Here's how the part is built. I have some questions about the finished solid (model axes, mm). A direction names the side the tool comes from. Coordinates: 2 decimals unless noted, no trailing zeros. Order: outer loops, then holes, each group sorted by start corner. A loop starts at its lowest first (then second) coordinate and runs counter-clockwise, first axis right, second up. Notation, with made-up numbers: (52.5, -37.75) - (91.5, -37.75) arc R8 cw to (91.5, -22.75) - close; hole circle Ø11 at (15, -1.75). An arc over 180 degrees is marked (long way). Use one line per item in the form item = value. Start each with the question number.
from build123d import *

# Parameters (mm, degrees)
SKETCH_1_W          = 55
SKETCH_1_H          = 55
EXTRUDE_1_DEPTH     = 10
EXTRUDE_2_DEPTH     = 55
CUT_EXTRUDE_1_DEPTH = 50
SKETCH_4_R          = 3
CUT_EXTRUDE_2_DEPTH = 10
SKETCH_5_R          = 1.5
CUT_EXTRUDE_3_DEPTH = 30


with BuildPart() as part:
    # 草图1 → 凸台-拉伸1 (new body)
    with BuildSketch(Plane.XY):
        Rectangle(SKETCH_1_W, SKETCH_1_H)
    extrude(amount=EXTRUDE_1_DEPTH)

    # 草图2 → 凸台-拉伸2 (add)
    with BuildSketch(Plane(origin=(27.5, 0, 0), x_dir=(0, 0, -1), z_dir=(1, 0, 0))):
        Polygon((0, -27.5), (-14.219889521, -52.26914509), (-61.918339647, -24.885612528), (-10, 27.5), align=None)
    extrude(amount=-EXTRUDE_2_DEPTH)

    # 草图3 → 切除-拉伸1 (cut)
    with BuildSketch(Plane(origin=(0, 0, 10), x_dir=(-1, 0, 0), z_dir=(0, 0, -1))):
        Polygon((22.5, 22.5), (22.5, -22.5), (-22.5, -22.5), (-22.5, 22.5), (-22.5, 36.625124929), (22.5, 36.625124929), align=None)
    extrude(amount=-CUT_EXTRUDE_1_DEPTH, mode=Mode.SUBTRACT)

    # 草图4 → 切除-拉伸2 (cut)
    with BuildSketch(Plane(origin=(0, 0, 0), x_dir=(-1, 0, 0), z_dir=(0, 0, -1))):
        with Locations((16, 0)):
            Circle(SKETCH_4_R)
        with Locations((11.313708499, -11.313708499)):
            Circle(SKETCH_4_R)
        with Locations((0, -16)):
            Circle(SKETCH_4_R)
        with Locations((-11.313708499, -11.313708499)):
            Circle(SKETCH_4_R)
        with Locations((-16, 0)):
            Circle(SKETCH_4_R)
        with Locations((-11.313708499, 11.313708499)):
            Circle(SKETCH_4_R)
        with Locations((0, 16)):
            Circle(SKETCH_4_R)
        with Locations((11.313708499, 11.313708499)):
            Circle(SKETCH_4_R)
    extrude(amount=-CUT_EXTRUDE_2_DEPTH, mode=Mode.SUBTRACT)

    # 草图5 → 切除-拉伸3 (cut)
    with BuildSketch(Plane(origin=(0, -45.452255494, 26.093999177), x_dir=(1, 0, 0), z_dir=(0, -0.8672445477434421, 0.4978824102228085))):
        with Locations(Location((10, 23.808233719, 0), (0, 0, 270))):
            Circle(SKETCH_5_R)
        with Locations(Location((10, 13.808233719, 0), (0, 0, 270))):
            Circle(SKETCH_5_R)
        with Locations(Location((0, 23.808233719, 0), (0, 0, 270))):
            Circle(SKETCH_5_R)
        with Locations(Location((-10, 23.808233719, 0), (0, 0, 90))):
            Circle(SKETCH_5_R)
        with Locations(Location((-10, 13.808233719, 0), (0, 0, 90))):
            Circle(SKETCH_5_R)
        with Locations(Location((-10, 3.808233719, 0), (0, 0, 270))):
            Circle(SKETCH_5_R)
        with Locations(Location((0, 3.808233719, 0), (0, 0, 90))):
            Circle(SKETCH_5_R)
        with Locations(Location((10, 3.808233719, 0), (0, 0, 90))):
            Circle(SKETCH_5_R)
    extrude(amount=-CUT_EXTRUDE_3_DEPTH, mode=Mode.SUBTRACT)


solid = part.part
1) Which directions (+Z, -Z, +X, -X, +Y, -Y) give clear straight access to the entire face, cutting with the end or side of a thin tool? Please do faces 1 (the flat face through (0, 3, 10)), 2 (the cylindrical face through (-10.575, -33.497, 22.024)).
2) For pin 1 (9.5 mm diameter, centred on x = 0, y = -16, fed in from +Z); pin 2 (8 mm diameter, centred on x = -11, z = 29.5, fed in from -Y); pin 3 (6 mm diameter, centred on x = 8.5, z = 32, fed in from +Y), each with a flat end and sliding along its axis, tell me the tip position at first contact or that it passes through.
3) I need wall thicknesses on probe 1 along X at (y, z) = (-7, 17); probe 2 along Y at (x, z) = (2, 8.5); probe 3 along Z at (x, y) = (-5.5, -9). Which ranges of each line are inside material? Lowest first, please. Write a range as [from, to].
4) Suppose I cut it at B-B, the plane x = -16. List the corners of the cut face in (y, z) for me, then the cut area to 3 significant figures.
5) If we mould it in two halves opening along Y, with no side actions, what happens to faces 3 (the flat face through (0.385, -38.769, 37.735)), 4 (the flat face through (22.5, -8, 23)), 5 (the cylindrical face through (-10.07, -28.47, 42.07))? For each: pulls with the +Y half, pulls with the -Y half, needs draft (parallel to the pull), parting line crosses it, or undercut.
6) Suppose I cut it at A-A, the plane y = 0. List the corners of the cut face in (x, z) for me.
7) Suppose I cut it at D-D, the plane x = 0. List the corners of the cut face in (y, z) for me, then the cut area to 3 significant figures.
8) Suppose I cut it at C-C, the plane y = 16. List the corners of the cut face in (x, z) for me.
From the geometry:
q1.face_1 = +Z, +Y
q1.face_2 = none
q2.pin_1 = 10
q2.pin_2 = -45.79
q2.pin_3 = -22.5
q3.probe_1 = [-27.5, -22.5], [22.5, 27.5]
q3.probe_2 = [-42.31, -18.24], [-13.76, 13.76], [18.24, 27.5]
q3.probe_3 = [0, 10]
q4.outline = (-52.27, 14.22) - (-27.5, 0) - (-3, 0) - (-3, 10) - (-22.5, 10) - (-22.5, 59.55) - (-24.89, 61.92) - close; (3, 0) - (27.5, 0) - (27.5, 10) - (3, 10) - close
q4.area = 1,450 mm2
q5.face_3 = pulls with the -Y half
q5.face_4 = needs draft
q5.face_5 = undercut
q6.outline = (-27.5, 0) - (-19, 0) - (-19, 10) - (-22.5, 10) - (-22.5, 37.25) - (-27.5, 37.25) - close; (-13, 0) - (13, 0) - (13, 10) - (-13, 10) - close; (19, 0) - (27.5, 0) - (27.5, 37.25) - (22.5, 37.25) - (22.5, 10) - (19, 10) - close
q7.outline = (-52.27, 14.22) - (-27.5, 0) - (-19, 0) - (-19, 10) - (-22.5, 10) - (-22.5, 15.58) - (-44.3, 28.1) - close; (-42.81, 30.7) - (-22.5, 19.04) - (-22.5, 38.64) - (-34.35, 45.44) - close; (-32.85, 48.04) - (-22.5, 42.1) - (-22.5, 59.55) - (-24.89, 61.92) - close; (-13, 0) - (13, 0) - (13, 10) - (-13, 10) - close; (19, 0) - (27.5, 0) - (27.5, 10) - (19, 10) - close
q7.area = 1,280 mm2
q8.outline = (-27.5, 0) - (-3, 0) - (-3, 10) - (-22.5, 10) - (-22.5, 21.4) - (-27.5, 21.4) - close; (3, 0) - (27.5, 0) - (27.5, 21.4) - (22.5, 21.4) - (22.5, 10) - (3, 10) - close
